Can you work these out from the model? Positions are in its coordinate system, mm. Face numbers are marked on the shaded views. Give positions to 0.01 mm unless a question says otherwise; leave off trailing zeros. Loops run counter-clockwise (first coordinate to the right, second up) from the corner with the lowest first, then second, coordinate; pieces in that order, holes last. Notation, with made-up numbers: (-38.75, -15.75) -> (-17.75, -15.75) arc R22 cw to (-17.75, 18.25) -> close; hole circle Ø5 at (-4, -1). An arc over 180 degrees is marked (long way). Use CSV: the item, a comma, the result in double quotes.
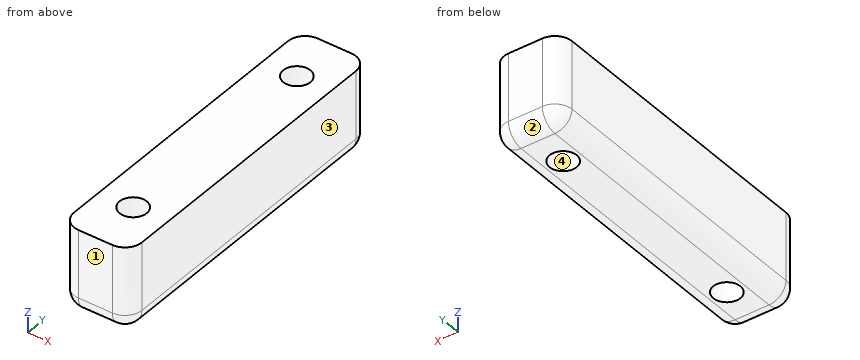
from build123d import *

# Parameters (mm, degrees)
CYLINDER051_R          = 0.8
CYLINDER051_DEPTH      = 10
CYLINDER050_R          = 0.8
CYLINDER050_DEPTH      = 10
CYLINDER047_R          = 0.75
CYLINDER047_DEPTH      = 10
CYLINDER046_R          = 0.75
CYLINDER046_DEPTH      = 10
BOX020_W               = 4
BOX020_H               = 19
BOX020_DEPTH           = 5
FILLET008_R            = 1
FILLET009_R            = 1
FILLET010_R            = 1
FILLET011_R            = 1
CUT066_PLACEMENT_ANGLE = 180


with BuildPart() as cilindro051:
    # Cylinder051 → Cylinder051 (new body)
    with BuildSketch(Plane(origin=(11, -17, -17), x_dir=(1, 0, 0), z_dir=(0, 0, 1))):
        Circle(CYLINDER051_R)
    extrude(amount=CYLINDER051_DEPTH)


with BuildPart() as cilindro050:
    # Cylinder050 → Cylinder050 (new body)
    with BuildSketch(Plane(origin=(11, -4, -17), x_dir=(1, 0, 0), z_dir=(0, 0, 1))):
        Circle(CYLINDER050_R)
    extrude(amount=CYLINDER050_DEPTH)


with BuildPart() as cilindro047:
    # Cylinder047 → Cylinder047 (new body)
    with BuildSketch(Plane(origin=(-39, 66, 48), x_dir=(1, 0, 0), z_dir=(0, 0, 1))):
        Circle(CYLINDER047_R)
    extrude(amount=CYLINDER047_DEPTH)


with BuildPart() as cilindro046:
    # Cylinder046 → Cylinder046 (new body)
    with BuildSketch(Plane(origin=(-39, 53, 48), x_dir=(1, 0, 0), z_dir=(0, 0, 1))):
        Circle(CYLINDER046_R)
    extrude(amount=CYLINDER046_DEPTH)


with BuildPart() as cut070:
    # Box020 → Box020 (new body)
    with BuildSketch(Plane(origin=(-2, 50, 45), x_dir=(1, 0, 0), z_dir=(0, 0, 1))):
        with Locations((2, 9.5)):
            Rectangle(BOX020_W, BOX020_H)
    extrude(amount=BOX020_DEPTH)

    # Fillet008
    fillet008_edges = [cut070.edges().sort_by_distance(p)[0] for p in [
        (2, 59.5, 50),
    ]]
    fillet(fillet008_edges, radius=FILLET008_R)

    # Fillet009
    fillet009_edges = [cut070.edges().sort_by_distance(p)[0] for p in [
        (-2, 59.5, 50),
    ]]
    fillet(fillet009_edges, radius=FILLET009_R)

    # Fillet010
    fillet010_edges = [cut070.edges().sort_by_distance(p)[0] for p in [
        (0, 69, 50),
    ]]
    fillet(fillet010_edges, radius=FILLET010_R)

    # Fillet011
    fillet011_edges = [cut070.edges().sort_by_distance(p)[0] for p in [
        (0, 50, 50),
    ]]
    fillet(fillet011_edges, radius=FILLET011_R)


with BuildPart() as cut070_1:
    # Fillet011 placement: moved
    add(cut070.part.moved(Location((-39, 0, 0))))

    # Cut065: cut Cilindro046
    add(cilindro046.part, mode=Mode.SUBTRACT)

    # Cut066: cut Cilindro047
    add(cilindro047.part, mode=Mode.SUBTRACT)


with BuildPart() as cut070_2:
    # Cut066 placement: moved
    add(cut070_1.part.moved(Location((-28, -70, 35))).rotate(Axis((-28, -70, 35), (0, 1, 0)), CUT066_PLACEMENT_ANGLE))

    # Cut069: cut Cilindro050
    add(cilindro050.part, mode=Mode.SUBTRACT)

    # Cut070: cut Cilindro051
    add(cilindro051.part, mode=Mode.SUBTRACT)


solid = cut070_2.part
(1) If we section it at D-D, the plane y = -10.5: Write out the boundary of the cut face in (x, z), then the cut area to 3 significant figures.
Answer sheet:
outline,"(9, -14) arc R1 ccw to (10, -15) -> (12, -15) arc R1 ccw to (13, -14) -> (13, -10) -> (9, -10) -> close"
area,"19.6 mm2"
(2) If we section it at A-A, the plane x = 11: Write out the boundary of the cut face in (y, z).
Answer sheet:
outline,"(-20, -14) arc R1 ccw to (-19, -15) -> (-17.8, -15) -> (-17.8, -10) -> (-20, -10) -> close; (-16.2, -15) -> (-4.8, -15) -> (-4.8, -10) -> (-16.2, -10) -> close; (-3.2, -15) -> (-2, -15) arc R1 ccw to (-1, -14) -> (-1, -10) -> (-3.2, -10) -> close"
(3) If we section it at B-B, the plane z = -12.4: Write out the boundary of the cut face in (x, y).
Answer sheet:
outline,"(9, -19) arc R1 ccw to (10, -20) -> (12, -20) arc R1 ccw to (13, -19) -> (13, -2) arc R1 ccw to (12, -1) -> (10, -1) arc R1 ccw to (9, -2) -> close; hole circle Ø1.6 at (11, -17); hole circle Ø1.6 at (11, -4)"
(4) If we section it at C-C, the plane y = -17: Write out the boundary of the cut face in (x, z), then the cut area to 3 significant figures.
Answer sheet:
outline,"(9, -14) arc R1 ccw to (10, -15) -> (10.2, -15) -> (10.2, -10) -> (9, -10) -> close; (11.8, -15) -> (12, -15) arc R1 ccw to (13, -14) -> (13, -10) -> (11.8, -10) -> close"
area,"11.6 mm2"
(5) If I drill on L1, parallel to Y at x = 11, z = -11.05; L2, parallel to Y at x = 11.7, z = -12.7; L3, parallel to X at y = -4, z = -11.75, over which ranges is the centre line in solid material (lowest first)? Write a range as from..to.
Answer sheet:
L1,"y = -20..-17.8, -16.2..-4.8, -3.2..-1"
L2,"y = -20..-17.39, -16.61..-4.39, -3.61..-1"
L3,"x = 9..10.2, 11.8..13"
(6) We'd pull the mould along Y, two halves only. Please class the marked faces 1, 2, 3 and 4: released by +Y, released by -Y, zero draft, split by the parting line, or undercut.
Answer sheet:
face 1,"released by -Y"
face 2,"released by +Y"
face 3,"zero draft"
face 4,"undercut"
